from build123d import *

# Parameters (mm, degrees)
F1_DEPTH = 38.1
F2_W     = 63.5
F2_H     = 3.175
F3_DEPTH = 44.451
F5_D     = 5.1054
F5_DEPTH = 12.7
F5_TIP   = 1.5338169022
F7_ANGLE = 180


with BuildPart() as f1:
    # F0 (on Front) → F1 (new body, symmetric)
    with BuildSketch(Plane.XZ):
        Polygon((0, 12.7), (0, 0), (44.45, 0), (44.45, 34.925), (22.225, 34.925), align=None)
    extrude(amount=F1_DEPTH, both=True)

    # F2 (on face) → F3 (cut, through all)
    with BuildSketch(Plane(origin=(0, 0, 0), x_dir=(0, -1, 0), z_dir=(-1, 0, 0))):
        with Locations((0, 1.5875)):
            Rectangle(F2_W, F2_H)
    extrude(amount=-F3_DEPTH, mode=Mode.SUBTRACT)

    # F5
    with Locations(Plane.YZ.offset(44.45)):
        with Locations((-22.225, 19.05), (22.225, 19.05)):
            Hole(F5_D / 2, depth=F5_DEPTH)
            with Locations((0, 0, -(F5_DEPTH + F5_TIP / 2))):  # 118° drill point
                Cone(0, F5_D / 2, F5_TIP, mode=Mode.SUBTRACT)

    # F6 (on face) → F7 (revolve, cut)
    with BuildSketch(Plane(origin=(-6.35, 0, 6.35), x_dir=(0, -1, 0), z_dir=(-0.7071067812, 0, 0.7071067812))):
        with BuildLine():
            Line((0, 11.8361525448), (0, 37.2361525448))
            ThreePointArc((0, 37.2361525448), (-12.7, 24.5361525448), (0, 11.8361525448))
        make_face()
    revolve(axis=Axis((10.9996798487, 0, 23.6996798487), (-0.7071067812, 0, -0.7071067812)), revolution_arc=F7_ANGLE, mode=Mode.SUBTRACT)


solid = f1.part
Verification items for the finished model (mm, model axes). A direction names the side the tool comes from. Coordinates: 2 decimals unless noted, no trailing zeros. Order: outer loops, then holes, each group sorted by start corner. A loop starts at its lowest first (then second) coordinate and runs counter-clockwise, first axis right, second up. Notation, with made-up numbers: M 16.25,-1 L 31.25,-1 A28 cw 31.25,23 Z; hole C 66,-13.5 d1. An arc over 180 degrees is marked long. Return JSON: item names as keys, results as strings.
1) Cross-section at D-D, the plane y = -3. Record the boundary of the cut face in (x, z) (3 decimals).
Answer list:
{"outline": "M 0,3.175 L 44.45,3.175 L 44.45,34.925 L 22.225,34.925 L 19.726,32.426 A12.341 cw 2.274,14.974 L 0,12.7 Z"}
2) Cross-section at C-C, the plane z = 29.5. Record the boundary of the cut face in (x, y).
Answer list:
{"outline": "M 16.8,-38.1 L 44.45,-38.1 L 44.45,38.1 L 16.8,38.1 L 16.8,9.7 A11.3 cw 16.8,-9.7 Z"}
3) Gauge pin test, flat ends, axial feed: pin 1 (4.5 mm diameter, centred on y = 22.225, z = 19.05, fed in from -X); pin 2 (4 mm diameter, centred on y = -22.225, z = 19.05, fed in from -X); pin 3 (4 mm diameter, centred on x = 15.5, y = 9, fed in from +Z). Record the tip position at first contact, or that the pin passes through.
Answer list:
{"pin 1": "x = 4.1", "pin 2": "x = 4.35", "pin 3": "z = 30.2"}
4) Cross-section at A-A, the plane y = 14. Record the boundary of the cut face in (x, z) (3 decimals).
Answer list:
{"outline": "M 0,3.175 L 44.45,3.175 L 44.45,34.925 L 22.225,34.925 L 0,12.7 Z"}
5) Thickness scan on L1, parallel to Y at x = 35.5, z = 19.05; L2, parallel to Z at x = 11, y = 17.5 (3 decimals); L3, parallel to Z at x = 32.5, y = 16.5 (3 decimals). Record the ranges inside material, lowest first. Write a range as [from, to].
Answer list:
{"L1": "[-38.1, -24.78], [-19.67, 19.67], [24.78, 38.1]", "L2": "[3.175, 23.7]", "L3": "[3.175, 34.925]"}
6) Access from +Z, -Z, +X, -X, +Y, -Y to the whole of each face (thin tool, end or side, straight path). Record for faces 1 (the flat face through (33, -1, 34.925)), 2 (the cylindrical face through (38.01, 22.78, 16.56)), 3 (the flat face through (22, -31.75, 2)).
Answer list:
{"face 1": "+Z, +X, -X, +Y, -Y", "face 2": "+X", "face 3": "-Z, +X, -X"}
7) Cross-section at B-B, the plane x = 3.5. Record the boundary of the cut face in (y, z) (3 decimals), and give its area (3 significant figures).
Answer list:
{"outline": "M -38.1,0 L -31.75,0 L -31.75,3.175 L 31.75,3.175 L 31.75,0 L 38.1,0 L 38.1,16.2 L 6.986,16.2 A10.249 cw -6.986,16.2 L -38.1,16.2 Z", "area": "1,010 mm2"}
8) Release check for a two-part mould opening along Y. For faces 4 (the flat face through (27, -38.1, 18)), 5 (the conical face through (30.48, -22.32, 18.62)), 6 (the flat face through (0, -1, 8)), 7 (the flat face through (27, 38.1, 18)) record: +Y half, -Y half, draft (parallel to the pull), parting line (faces both ways), or undercut.
Answer list:
{"face 4": "-Y half", "face 5": "undercut", "face 6": "draft", "face 7": "+Y half"}
